```python
from build123d import *

# Parameters (mm, degrees)
F0_W     = 1.5
F0_H     = 1.5
F0_H_2   = 23.5
F0_W_2   = 23.5
F1_DEPTH = 84
F3_DEPTH = 25


with BuildPart() as f1:
    # F0 (on Top) → F1 (new body)
    with BuildSketch(Plane.XY):
        with Locations((11.75, 0)):
            Rectangle(F0_W, F0_H)
        with Locations((11.75, 12.5)):
            Rectangle(F0_W, F0_H_2)
        with Locations((-0.75, 0)):
            Rectangle(F0_W_2, F0_H)
    extrude(amount=-F1_DEPTH)

    # F2 (on face) → F3 (cut)
    with BuildSketch(Plane.XZ.offset(0.75)):
        Polygon((-12.5, -84), (12.5, -84), (-12.5, -37.333333), align=None)
    extrude(amount=-F3_DEPTH, mode=Mode.SUBTRACT)


solid = f1.part
```
The listing builds one solid part. Answer for the finished solid, in the listing's coordinates (mm). A direction names the side the tool comes from. Coordinates: 2 decimals unless noted, no trailing zeros. Loops run counter-clockwise (first coordinate to the right, second up) from the corner with the lowest first, then second, coordinate; pieces in that order, holes last. Notation, with made-up numbers: (-12.75, 20) -> (23.25, 20) arc R10 cw to (23.25, 36) -> close; hole circle Ø5 at (40, -36). An arc over 180 degrees is marked (long way). Return JSON: item names as keys, results as strings. Group by question number.
(1) Which of the six approach directions +Z, -Z, +X, -X, +Y, -Y give full straight-line access (tool end or side, diameter ignored) to faces 1 (the flat face through (11, 13, -40)), 2 (the flat face through (3, -0.75, -32))?
(2) Find the intervals of material crossed by probe 1 along Y at (x, z) = (9.25, -50.5); probe 2 along X at (y, z) = (20, -37), in increasing order. Write a range as from..to.
(3) A cutting plane is placed at B-B on y = 22. Write down the section's boundary in (x, z), and give its area (3 significant figures).
(4) A cutting plane is placed at D-D on z = -19.5. Write down the section's boundary in (x, y), and give its area (4 significant figures).
(5) A cutting plane is placed at C-C on z = -57. Write down the section's boundary in (x, y).
(6) Given pin 1 Ø1.5 at (y, z) = (12, -57) entering from -X; pin 2 Ø1.5 at (x, z) = (3, -11) entering from +Y, each flat-ended and moving along its own axis, determine where each tip first touches the part or whether it passes through.
(7) A cutting plane is placed at A-A on x = 0.5. Write down the section's boundary in (y, z), and give its area (3 significant figures).
The answers:
{
 "1": {"face 1": "+Z, -Z, -X, +Y", "face 2": "+Z, -Z, +X, -X, -Y"},
 "2": {"probe 1": "y = -0.75..0.75", "probe 2": "x = 11..12.5"},
 "3": {"outline": "(11, -81.2) -> (12.5, -84) -> (12.5, 0) -> (11, 0) -> close", "area": "124 mm^2"},
 "4": {"outline": "(-12.5, -0.75) -> (12.5, -0.75) -> (12.5, 24.25) -> (11, 24.25) -> (11, 0.75) -> (-12.5, 0.75) -> close", "area": "72.75 mm^2"},
 "5": {"outline": "(-1.96, -0.75) -> (12.5, -0.75) -> (12.5, 24.25) -> (11, 24.25) -> (11, 0.75) -> (-1.96, 0.75) -> close"},
 "6": {"pin 1": "stops at x = 11", "pin 2": "stops at y = 0.75"},
 "7": {"outline": "(-0.75, -61.6) -> (0.75, -61.6) -> (0.75, 0) -> (-0.75, 0) -> close", "area": "92.4 mm^2"}
}
